Can you work these out from the model? Positions are in its coordinate system, mm. A direction names the side the tool comes from. Coordinates: 2 decimals unless noted, no trailing zeros. Order: outer loops, then holes, each group sorted by start corner. A loop starts at its lowest first (then second) coordinate and runs counter-clockwise, first axis right, second up. Notation, with made-up numbers: (42.5, 2) -> (86.5, 2) arc R4 ccw to (86.5, 8) -> close; hole circle Ø8 at (-3.75, 61). An arc over 180 degrees is marked (long way). Answer in a Markdown table with one row per item.
```python
from build123d import *

# Parameters (mm, degrees)
BOSS_EXTRUDE1_DEPTH   = 6.35
F_6_32_TAPPED_HOLE2_D = 2.7051
F_6_32_TAPPED_HOLE1_D = 2.7051


with BuildPart() as part:
    # Sketch1 → Boss-Extrude1 (new body)
    with BuildSketch(Plane.XY):
        with BuildLine():
            Line((-30.725, 12.7), (-30.725, 10.16))
            Line((-30.725, 10.16), (-28.99655195, 10.16))
            ThreePointArc((-28.99655195, 10.16), (-28.338337344, 11.872837132), (-27.579048351, 13.5433274))
            ThreePointArc((-27.579048351, 13.5433274), (-29.797475058, 24.232437752), (-40.703834208, 24.711840767))
            ThreePointArc((-40.703834208, 24.711840767), (-44.411023794, 22.861749744), (-48.505, 22.225))
            Line((-48.505, 22.225), (-60.8875, 22.225))
            ThreePointArc((-60.8875, 22.225), (-70.990288136, 18.040288136), (-75.175, 7.9375))
            Line((-75.175, 7.9375), (-75.175, -7.9375))
            ThreePointArc((-75.175, -7.9375), (-73.061327111, -16.658929011), (-67.189349187, -23.445003896))
            ThreePointArc((-67.189349187, -23.445003896), (-44.21739693, -36.463267178), (-19.05, -44.45))
            Line((-19.05, -44.45), (0, -44.45))
            Line((0, -44.45), (0, -30.725))
            ThreePointArc((0, -30.725), (-17.774414547, -25.061839767), (-28.99655195, -10.16))
            Line((-28.99655195, -10.16), (-30.725, -10.16))
            Line((-30.725, -10.16), (-30.725, -12.7))
            ThreePointArc((-30.725, -12.7), (-33.481957403, -17.019630209), (-38.560886674, -16.338090241))
            ThreePointArc((-38.560886674, -16.338090241), (-43.210637658, -13.638076264), (-48.505, -12.7))
            Line((-48.505, -12.7), (-56.125, -12.7))
            ThreePointArc((-56.125, -12.7), (-59.492596045, -11.305096045), (-60.8875, -7.9375))
            Line((-60.8875, -7.9375), (-60.8875, 7.9375))
            ThreePointArc((-60.8875, 7.9375), (-59.492596045, 11.305096045), (-56.125, 12.7))
            Line((-56.125, 12.7), (-48.505, 12.7))
            ThreePointArc((-48.505, 12.7), (-43.210637658, 13.638076264), (-38.560886674, 16.338090241))
            ThreePointArc((-38.560886674, 16.338090241), (-33.481957403, 17.019630209), (-30.725, 12.7))
        make_face()
    boss_extrude1 = extrude(amount=BOSS_EXTRUDE1_DEPTH)

    # Mirror1: Boss-Extrude1 across plane
    add(boss_extrude1.mirror(Plane(origin=(0, -30.725, 6.35), x_dir=(0, 0, 1), z_dir=(-1, 0, 0))))

    # #6-32 Tapped Hole2 (through all)
    with Locations(Plane(origin=(0, -44.45, 0), x_dir=(-1, 0, 0), z_dir=(0, -1, 0))):
        with Locations((-12.7, -3.175), (12.7, -3.175)):
            Hole(F_6_32_TAPPED_HOLE2_D / 2)

    # #6-32 Tapped Hole1 (through all)
    with Locations(Plane.ZY.offset(75.175)):
        with Locations((3.175, 0)):
            Hole(F_6_32_TAPPED_HOLE1_D / 2)


solid = part.part
```
(1) On a 3-axis mill with a long thin cutter (end or side, diameter ignored), from which of +Z, -Z, +X, -X, +Y, -Y can I reach the whole of each face in a straight line? I mean faces 5 (the cylindrical face through (33.414, -16.987, 3.131)), 6 (the cylindrical face through (-67.931, 0.059, 4.526)). Say none if no direction works.
Response values:
| item | result |
|---|---|
| face 5 | +Z, -Z |
| face 6 | +X, -X |
(2) Suppose I cut it at C-C (x = 12.7). Please give me the cut outline in (y, z), and give its area (3 significant figures).
Response values:
| item | result |
|---|---|
| outline | (-44.45, 0) -> (-27.98, 0) -> (-27.98, 1.82) -> (-44.45, 1.82) -> close; (-44.45, 4.53) -> (-27.98, 4.53) -> (-27.98, 6.35) -> (-44.45, 6.35) -> close |
| area | 60.0 mm2 |
(3) I need wall thicknesses on line 1 (X direction, y = -7.5, z = 0.5) (1 decimal); line 2 (X direction, y = -17, z = 3); line 3 (X direction, y = 15, z = 4.75). Which ranges of each line are inside material? Lowest first, please. Write a range as [from, to].
Response values:
| item | result |
|---|---|
| line 1 | [-75.2, -60.9], [60.9, 75.2] |
| line 2 | [-72.88, -37.53], [-33.44, -25.59], [25.59, 33.44], [37.53, 72.88] |
| line 3 | [-73.31, -40.41], [-31.32, -27.02], [27.02, 31.32], [40.41, 73.31] |
(4) We'd pull the mould along X, two halves only. Please class faces 1 (the cylindrical face through (-59.5, 11.3, 3.1)), 2 (the flat face through (-75.175, 0, 5)), 3 (the flat face through (55, 22.225, 3)), 4 (the flat face through (-30.725, -11, 3)): +X half, -X half, draft (parallel to the pull), parting line (faces both ways), or undercut.
Response values:
| item | result |
|---|---|
| face 1 | undercut |
| face 2 | -X half |
| face 3 | draft |
| face 4 | undercut |
(5) Will these pins go through, and if not, where does the flat tip stop? pin 1 Ø3 at (x, z) = (-43, 5) entering from +Y; pin 2 Ø3 at (x, z) = (-31.5, 4.5) entering from -Y; pin 3 Ø1.9 at (x, z) = (-29.5, 3) entering from -Y.
Response values:
| item | result |
|---|---|
| pin 1 | y = 24.19 |
| pin 2 | y = -41.68 |
| pin 3 | y = -42.11 |
(6) Suppose I cut it at B-B (y = -22). Please give me the cut outline in (x, z), and give its area (3 significant figures).
Response values:
| item | result |
|---|---|
| outline | (-68.98, 0) -> (-21.45, 0) -> (-21.45, 6.35) -> (-68.98, 6.35) -> close; (21.45, 0) -> (68.98, 0) -> (68.98, 6.35) -> (21.45, 6.35) -> close |
| area | 604 mm2 |
(7) Suppose I cut it at D-D (y = -34.5). Please give me the cut outline in (x, z) (3 decimals), and give its area (3 significant figures).
Response values:
| item | result |
|---|---|
| outline | (-48.498, 0) -> (48.498, 0) -> (48.498, 6.35) -> (-48.498, 6.35) -> close; hole circle Ø2.705 at (-12.7, 3.175); hole circle Ø2.705 at (12.7, 3.175) |
| area | 604 mm2 |
(8) Suppose I cut it at A-A (y = 0). Count the separate pieces of the cut face and the enclosed holes in it, and give its area (3 significant figures).
Response values:
| item | result |
|---|---|
| separate pieces | 4 |
| enclosed holes | 0 |
| area | 104 mm2 |
